from build123d import *

# Parameters (mm, degrees)
F1_DEPTH = 9.525
F3_DEPTH = 38.1
F4_R     = 2.2225
F5_DEPTH = 12.7
F6_R     = 5.08
F7_DEPTH = 9.525


with BuildPart() as f1:
    # F0 (on Top) → F1 (new body)
    with BuildSketch(Plane.XY):
        with BuildLine():
            Line((-10.16, -16.51), (-10.16, -6.35))
            Line((-10.16, -6.35), (0, -6.35))
            Line((0, -6.35), (0, -16.51))
            Line((0, -16.51), (12.7, -16.51))
            Line((12.7, -16.51), (12.7, -6.35))
            Line((12.7, -6.35), (12.7, 15.231052))
            Line((12.7, 15.231052), (-16.51, 15.231052))
            ThreePointArc((-16.51, 15.231052), (-18.755064, 14.301116), (-19.685, 12.056052))
            ThreePointArc((-19.685, 12.056052), (-18.755064, 9.810988), (-16.51, 8.881052))
            Line((-16.51, 8.881052), (-16.51, -16.51))
            Line((-16.51, -16.51), (-10.16, -16.51))
        make_face()
    extrude(amount=F1_DEPTH)

    # F2 (on face) → F3 (join)
    with BuildSketch(Plane.XY.offset(9.525)):
        with BuildLine():
            ThreePointArc((-16.51, 8.881052), (-14.264936, 9.810988), (-13.335, 12.056052))
            ThreePointArc((-13.335, 12.056052), (-14.264936, 14.301116), (-16.51, 15.231052))
            ThreePointArc((-16.51, 15.231052), (-19.685, 12.056052), (-16.51, 8.881052))
        make_face()
    extrude(amount=F3_DEPTH)

    # F4 (on face) → F5 (cut, through all)
    with BuildSketch(Plane.YZ.offset(12.7)):
        with Locations((-11.43, 4.7625)):
            Circle(F4_R)
    extrude(amount=-F5_DEPTH, mode=Mode.SUBTRACT)

    # F6
    f6_edges = [f1.edges().sort_by_distance(p)[0] for p in [
        (12.7, 15.231052, 4.7625),
    ]]
    fillet(f6_edges, radius=F6_R)

    # F0 (on Top) → F7 (join)
    with BuildSketch(Plane.XY):
        with BuildLine():
            Line((-19.685, -16.51), (-16.51, -16.51))
            Line((-16.51, -16.51), (-16.51, 8.881052))
            ThreePointArc((-16.51, 8.881052), (-18.755064, 9.810988), (-19.685, 12.056052))
            Line((-19.685, 12.056052), (-19.685, -16.51))
        make_face()
    extrude(amount=F7_DEPTH)


solid = f1.part
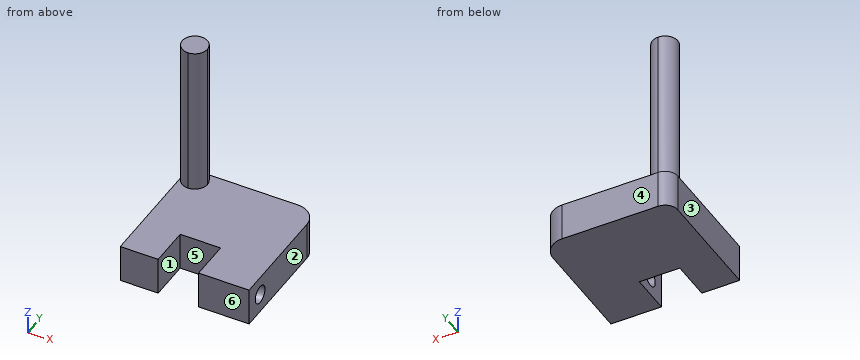
Geometry check sheet. Reference: the model listing, model coordinates, mm. Face numbers are marked on the shaded views. A direction names the side the tool comes from. Coordinates: 2 decimals unless noted, no trailing zeros. Write each loop counter-clockwise with the first axis right and the second up, starting at its lowest first coordinate (ties: lowest second). Pieces come first, ordered by that corner, then holes. Notation, with made-up numbers: (55, 70) -> (77, 70) arc R19 ccw to (77, 99) -> close; hole circle Ø4 at (2.5, -23.5). An arc over 180 degrees is marked (long way). One line per question, with ' | ' between items.
1. Thickness scan on probe 1 along Z at (x, y) = (9, -11.43) (3 decimals); probe 2 along Z at (x, y) = (10.5, 8) (3 decimals); probe 3 along Y at (x, z) = (-2.5, 4). Record the ranges inside material, lowest first. Write a range as from..to.
Answers:
probe 1: z = 0..2.54, 6.985..9.525 | probe 2: z = 0..9.525 | probe 3: y = -6.35..15.23
2. Cross-section at A-A on y = -11.43. Record the cut outline in (x, z) (3 decimals).
Answers:
outline: (-19.685, 0) -> (-10.16, 0) -> (-10.16, 9.525) -> (-19.685, 9.525) -> close; (0, 0) -> (12.7, 0) -> (12.7, 2.54) -> (0, 2.54) -> close; (0, 6.985) -> (12.7, 6.985) -> (12.7, 9.525) -> (0, 9.525) -> close
3. Depth check by flat-ended pin: pin 1 Ø7.5 at (x, z) = (-4, 5.5) entering from -Y; pin 2 Ø2 at (x, y) = (-4, 1) entering from +Z (3 decimals); pin 3 Ø2.5 at (y, z) = (-11.43, 4.76) entering from +X. Enter the tip coordinate at first touch or a pass-through.
Answers:
pin 1: stops at y = -6.35 | pin 2: stops at z = 9.525 | pin 3: stops at x = -10.16
4. Draft check along X on the marked faces 1, 2, 3 and 4. Enter one of: +X half, -X half, draft (parallel to the pull), parting line (faces both ways), or undercut.
Answers:
face 1: undercut | face 2: +X half | face 3: -X half | face 4: draft
5. Cross-section at D-D on z = 26.5. Record the cut outline in (x, y) (3 decimals).
Answers:
outline: circle Ø6.35 at (-16.51, 12.056)
6. Set-up check for the marked faces 5 and 6: record each of +Z, -Z, +X, -X, +Y, -Y from which the full face is reachable in a straight line by a thin tool's end or side.
Answers:
face 5: +Z, -Z, -Y | face 6: +Z, -Z, +X, -X, -Y
7. Cross-section at C-C on x = -2.5. Record the cut outline in (y, z) (3 decimals).
Answers:
outline: (-6.35, 0) -> (15.231, 0) -> (15.231, 9.525) -> (-6.35, 9.525) -> close
8. Cross-section at B-B on x = 9.5. Record the cut outline in (y, z) (1 decimal).
Answers:
outline: (-16.5, 0) -> (14.9, 0) -> (14.9, 9.5) -> (-16.5, 9.5) -> close; hole circle Ø4.4 at (-11.4, 4.8)
